```python
from build123d import *

# Parameters (mm, degrees)
SKETCH_1_R          = 70
EXTRUDE_1_DEPTH     = 8
CUT_EXTRUDE_1_DEPTH = 8
SKETCH_3_R          = 2
CUT_EXTRUDE_2_DEPTH = 8


with BuildPart() as part:
    # 草图1 → 凸台-拉伸1 (new body)
    with BuildSketch(Plane.XY):
        Circle(SKETCH_1_R)
    extrude(amount=EXTRUDE_1_DEPTH)

    # 草图2 → 切除-拉伸1 (cut)
    with BuildSketch(Plane.XY.offset(8)):
        with BuildLine():
            ThreePointArc((9.24720137, 57.806476957), (0, 64), (-9.24720137, 57.806476957))
            ThreePointArc((-9.24720137, 57.806476957), (-17.987701275, 49.420803081), (-30.073519924, 50.226316914))
            ThreePointArc((-30.073519924, 50.226316914), (-41.13840702, 49.02684436), (-44.241054371, 38.338343984))
            ThreePointArc((-44.241054371, 38.338343984), (-45.546458487, 26.296260068), (-55.322507015, 19.144704984))
            ThreePointArc((-55.322507015, 19.144704984), (-63.027696193, 11.113483371), (-58.534026348, 0.931273778))
            ThreePointArc((-58.534026348, 0.931273778), (-51.793521581, -9.132595281), (-54.685478233, -20.894927178))
            ThreePointArc((-54.685478233, -20.894927178), (-55.425625842, -32), (-45.438276863, -36.911549779))
            ThreePointArc((-45.438276863, -36.911549779), (-33.805820306, -40.2882078), (-28.460506424, -51.157590692))
            ThreePointArc((-28.460506424, -51.157590692), (-21.889289173, -60.14032773), (-11.081452644, -57.483048968))
            ThreePointArc((-11.081452644, -57.483048968), (0, -52.592520136), (11.081452644, -57.483048968))
            ThreePointArc((11.081452644, -57.483048968), (21.889289173, -60.14032773), (28.460506424, -51.157590692))
            ThreePointArc((28.460506424, -51.157590692), (33.805820306, -40.2882078), (45.438276863, -36.911549779))
            ThreePointArc((45.438276863, -36.911549779), (55.425625842, -32), (54.685478233, -20.894927178))
            ThreePointArc((54.685478233, -20.894927178), (51.793521581, -9.132595281), (58.534026348, 0.931273778))
            ThreePointArc((58.534026348, 0.931273778), (63.027696193, 11.113483371), (55.322507015, 19.144704984))
            ThreePointArc((55.322507015, 19.144704984), (45.546458487, 26.296260068), (44.241054371, 38.338343984))
            ThreePointArc((44.241054371, 38.338343984), (41.13840702, 49.02684436), (30.073519924, 50.226316914))
            ThreePointArc((30.073519924, 50.226316914), (17.987701275, 49.420803081), (9.24720137, 57.806476957))
        make_face()
    extrude(amount=-CUT_EXTRUDE_1_DEPTH, mode=Mode.SUBTRACT)

    # 草图3 → 切除-拉伸2 (cut)
    with BuildSketch(Plane(origin=(0, 0, 0), x_dir=(-1, 0, 0), z_dir=(0, 0, -1))):
        with Locations((21.205248886, 58.260942489)):
            Circle(SKETCH_3_R)
        with Locations((53.693575035, 31)):
            Circle(SKETCH_3_R)
        with Locations((61.058080687, -10.766187015)):
            Circle(SKETCH_3_R)
        with Locations((39.852831801, -47.494755473)):
            Circle(SKETCH_3_R)
        with Locations((0, -62)):
            Circle(SKETCH_3_R)
        with Locations((-39.852831801, -47.494755473)):
            Circle(SKETCH_3_R)
        with Locations((-61.058080687, -10.766187015)):
            Circle(SKETCH_3_R)
        with Locations((-53.693575035, 31)):
            Circle(SKETCH_3_R)
        with Locations((-21.205248886, 58.260942489)):
            Circle(SKETCH_3_R)
    extrude(amount=-CUT_EXTRUDE_2_DEPTH, mode=Mode.SUBTRACT)


solid = part.part
```
Input: part model. Units: mm. Frame: model coordinates. Round coordinates to 2 decimals unless told otherwise and drop trailing zeros. Loops run counter-clockwise (first coordinate to the right, second up) from the corner with the lowest first, then second, coordinate; pieces in that order, holes last. Notation, with made-up numbers: (25, 0) -> (72, 0) arc R20 ccw to (72, 36) -> close; hole circle Ø9 at (49.25, 8.25). An arc over 180 degrees is marked (long way). Write each question's results on one line, items separated by ' | '.
1. Ray query, line 1 (X direction, y = -49, z = 5.75); line 2 (Y direction, x = -60.5, z = 2.5); line 3 (X direction, y = 58, z = 5.5). Return the intervals inside material, ascending. Write a range as from..to.
Geometry results:
line 1: -49.99..-41.17, -38.54..-28.71, 28.71..38.54, 41.17..49.99 | line 2: -35.21..-12.69, -8.85..2.56, 16.19..35.21 | line 3: -39.19..-23.19, -19.22..-9.17, 9.17..19.22, 23.19..39.19
2. Section A-A (x = 0). Return loops of the section in (y, z), and give its area (3 significant figures).
Geometry results:
outline: (-70, 0) -> (-64, 0) -> (-64, 8) -> (-70, 8) -> close; (-60, 0) -> (-52.59, 0) -> (-52.59, 8) -> (-60, 8) -> close; (64, 0) -> (70, 0) -> (70, 8) -> (64, 8) -> close | area: 155 mm2
3. Section B-B (y = 31). Return loops of the section in (x, z).
Geometry results:
outline: (-62.76, 0) -> (-55.69, 0) -> (-55.69, 8) -> (-62.76, 8) -> close; (-51.69, 0) -> (-43.8, 0) -> (-43.8, 8) -> (-51.69, 8) -> close; (43.8, 0) -> (51.69, 0) -> (51.69, 8) -> (43.8, 8) -> close; (55.69, 0) -> (62.76, 0) -> (62.76, 8) -> (55.69, 8) -> close
4. Mould query, pull axis X, two halves, no side actions, for faces 1 (the face through (55.342, -32.142, 4.056)), 2 (the face through (-55.55, -42.594, 3.944)). Classes: +X half, -X half, draft (parallel to the pull), parting line (faces both ways), or undercut.
Geometry results:
face 1: undercut | face 2: parting line
5. Section C-C (x = 15.5). Return loops of the section in (y, z).
Geometry results:
outline: (-68.26, 0) -> (-60.29, 0) -> (-60.29, 8) -> (-68.26, 8) -> close; (50.59, 0) -> (68.26, 0) -> (68.26, 8) -> (50.59, 8) -> close
6. First-contact query: P1, Ø1, axis at x = -15.5, z = 6, coming from the +Y side; P2, Ø1.5, axis at y = 20.5, z = 1.5, coming from the -X side; P3, Ø6.5, axis at x = -53.69, y = 31, coming from the +Z side; P4, Ø1, axis at x = -12.5, z = 6.5, coming from the -Y side. Flat tips, straight axial feed; report the tip coordinate or a pass-through.
Geometry results:
P1: y = 68.37 | P2: x = -67.16 | P3: z = 8 | P4: y = -68.96
7. Section D-D (z = 2). State how many separate pieces and enclosed holes the cut face has, and give its area (3 significant figures).
Geometry results:
separate pieces: 1 | enclosed holes: 10 | area: 4,670 mm2
